```python
from build123d import *

# Parameters (mm, degrees)
REDONDEO1_R = 2
REDONDEO2_R = 2
REDONDEO3_R = 1
REDONDEO4_R = 1


with BuildPart() as part:
    # Croquis1 → Revolución1 (revolve)
    with BuildSketch(Plane.XY):
        Polygon((-12.649708752, 0), (15.350291248, 0), (15.350291248, 8), (12.350291248, 8), (12.350291248, 28), (15.350291248, 28), (15.350291248, 43), (-12.649708752, 43), (-12.649708752, 28), (-9.649708752, 28), (-9.649708752, 8), (-12.649708752, 8), align=None)
    revolve(axis=Axis((-30.163665743, -7, 0), (1, 0, 0)))

    # Redondeo1
    redondeo1_edges = [part.edges().sort_by_distance(p)[0] for p in [
        (15.350291248, -57, 0),
    ]]
    fillet(redondeo1_edges, radius=REDONDEO1_R)

    # Redondeo2
    redondeo2_edges = [part.edges().sort_by_distance(p)[0] for p in [
        (-12.649708752, -57, 0),
    ]]
    fillet(redondeo2_edges, radius=REDONDEO2_R)

    # Redondeo3
    redondeo3_edges = [part.edges().sort_by_distance(p)[0] for p in [
        (-12.649708752, -42, 0),
    ]]
    fillet(redondeo3_edges, radius=REDONDEO3_R)

    # Redondeo4
    redondeo4_edges = [part.edges().sort_by_distance(p)[0] for p in [
        (15.350291248, -42, 0),
    ]]
    fillet(redondeo4_edges, radius=REDONDEO4_R)


solid = part.part
```
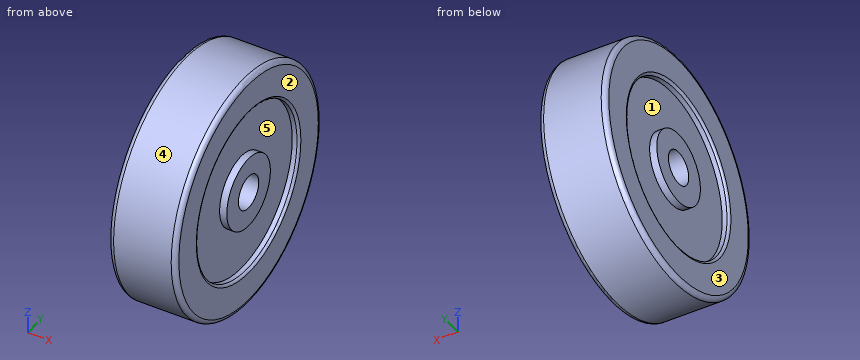
The listing builds one solid part. Answer for the finished solid, in the listing's coordinates (mm). Face numbers are marked on the shaded views. A direction names the side the tool comes from. Round coordinates to 2 decimals unless told otherwise and drop trailing zeros. Loops run counter-clockwise (first coordinate to the right, second up) from the corner with the lowest first, then second, coordinate; pieces in that order, holes last.
Q1. For a pull along Y with two mould halves and no side action, classify the marked faces 3, 4 and 5 as released by +Y, released by -Y, zero draft, split by the parting line, or undercut.
Q2. Find the intervals of material crossed by line 1 (Z direction, x = 13.4, y = -7); line 2 (Z direction, x = 4.5, y = -7); line 3 (X direction, y = -27, z = 19), in increasing order.
Q3. Section C-C, the plane x = 2.5 is taken. Determine the outline of the cut face in (y, z).
Q4. Which of the six approach directions +Z, -Z, +X, -X, +Y, -Y give full straight-line access (tool end or side, diameter ignored) to the marked faces 1 and 2?
Q5. Given pin 1 Ø4 at (x, y) = (9, -9) entering from -Z; pin 2 Ø8 at (x, y) = (0, -23.5) entering from -Z; pin 3 Ø4 at (x, y) = (4.5, 6.5) entering from -Z, each flat-ended and moving along its own axis, determine where each tip first touches the part or whether it passes through.
Completed:
1. face 3: zero draft
1. face 4: split by the parting line
1. face 5: undercut
2. line 1: z = -50 to -35, -15 to -7, 7 to 15, 35 to 50
2. line 2: z = -50 to -7, 7 to 50
2. line 3: x = -9.65 to 12.35
3. outline: circle Ø100 at (-7, 0); hole circle Ø14 at (-7, 0)
4. face 1: -X
4. face 2: +Z, -Z, +X, +Y, -Y
5. pin 1: stops at z = -50
5. pin 2: stops at z = -48.41
5. pin 3: stops at z = -48.66
